Input: dimensioned drawing with shaded views. Units: mm. Origin: part minimum x, y, z. Give positions to 0.01 mm unless a question says otherwise; leave off trailing zeros. Order: outer loops, then holes, each group sorted by start corner. A loop starts at its lowest first (then second) coordinate and runs counter-clockwise, first axis right, second up. Notation, with made-up numbers: (38.25, 51) -> (91.25, 51) arc R27 ccw to (91.25, 78) -> close; hole circle Ø6 at (9.25, -8.5). An arc over 180 degrees is marked (long way). One line per question, with ' | ' between items. Start each with the question number.
(1) Section D-D (z = 2.25). Return loops of the section in (x, y) (1 decimal).
(2) Section C-C (y = 0.6). State how many separate pieces and enclosed holes the cut face has, then the cut area to 3 significant figures.
(3) Section A-A (x = 1.75). Return loops of the section in (y, z) (1 decimal).
(4) Ray query, L1, parallel to X at y = 0.2, z = 9.5 (1 decimal); L2, parallel to Z at x = 3.25, y = 0.85 (1 decimal); L3, parallel to X at y = 0.9, z = 6.5. Return the intervals inside material, ascending.
(5) First-contact query: pin 1 Ø6 at (x, z) = (8.5, 13.5) entering from +Y; pin 2 Ø0.5 at (x, y) = (3.5, 0.5) entering from -Z (1 decimal). Flat tips, straight axial feed; report the tip coordinate or a pass-through.
(6) Section B-B (z = 9.75). Return loops of the section in (x, y) (1 decimal).
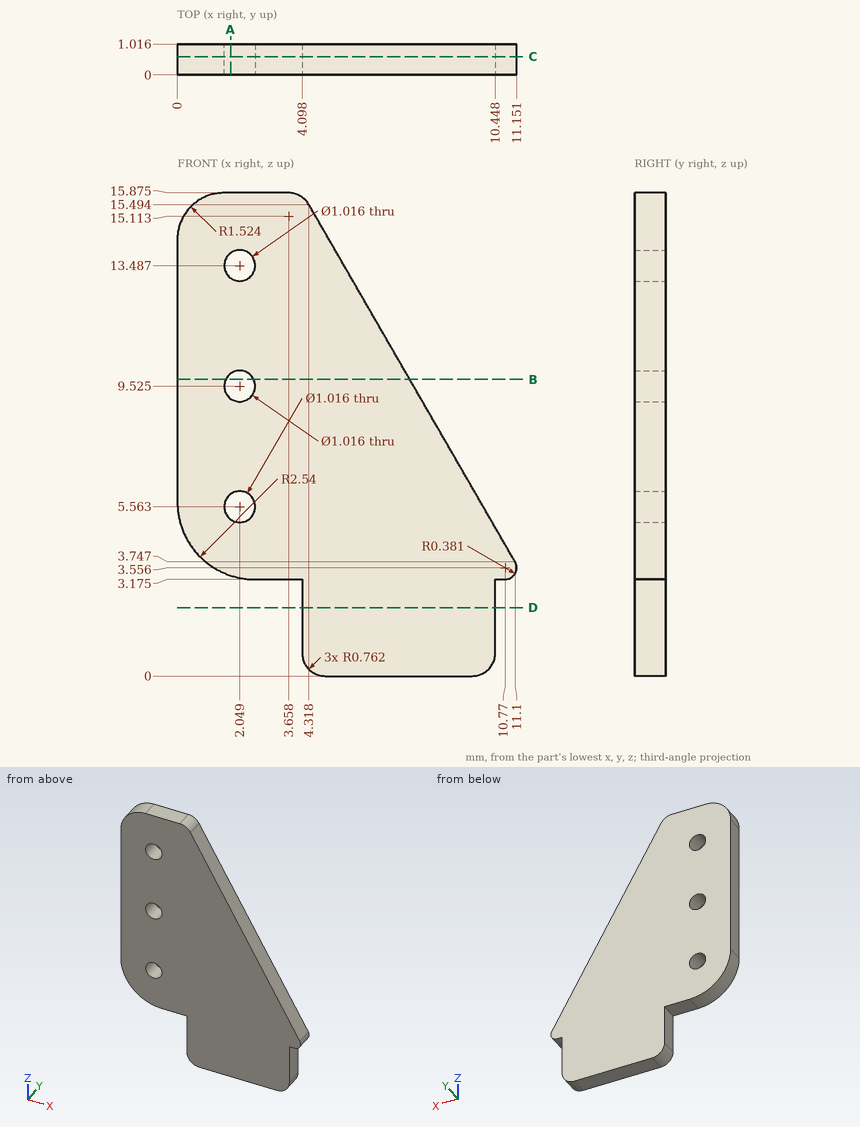
Response:
1) outline: (4.1, 0) -> (10.4, 0) -> (10.4, 1) -> (4.1, 1) -> close
2) separate pieces: 1 | enclosed holes: 3 | area: 114 mm^2
3) outline: (0, 3.3) -> (1, 3.3) -> (1, 5.2) -> (0, 5.2) -> close; (0, 6) -> (1, 6) -> (1, 9.1) -> (0, 9.1) -> close; (0, 9.9) -> (1, 9.9) -> (1, 13.1) -> (0, 13.1) -> close; (0, 13.9) -> (1, 13.9) -> (1, 15.9) -> (0, 15.9) -> close
4) L1: x = 0 to 1.5, 2.6 to 7.8 | L2: z = 3.2 to 15.9 | L3: x = 0 to 9.51
5) pin 1: stops at y = 1.02 | pin 2: stops at z = 3.2
6) outline: (0, 0) -> (1.6, 0) -> (1.6, 1) -> (0, 1) -> close; (2.5, 0) -> (7.6, 0) -> (7.6, 1) -> (2.5, 1) -> close
